The listing builds one solid part. Answer for the finished solid, in the listing's coordinates (mm). Coordinates: 2 decimals unless noted, no trailing zeros. Order: outer loops, then holes, each group sorted by start corner. A loop starts at its lowest first (then second) coordinate and runs counter-clockwise, first axis right, second up. Notation, with made-up numbers: (30.25, 54.5) - (81.25, 54.5) arc R17 cw to (81.25, 58.5) - close; hole circle Ø10 at (7.25, 23). An arc over 180 degrees is marked (long way). Use a Markdown table: item, result. Add a question column.
Item 1: The part is cut by section C-C, the plane x = 36. Give the vertices of the cut face in (y, z), then the cut area to 3 significant figures.
Item 2: The part is cut by section B-B, the plane x = 0. Give the vertices of the cut face in (y, z) (3 decimals).
Item 3: A flat-ended cylindrical pin translates along its axis: P1, Ø19, axis at x = 0, y = 0, coming from the -Z side. Find the tip coordinate at first contact, or state that the pin passes through.
Item 4: The part is cut by section A-A, the plane z = 0. Give the vertices of the cut face in (x, y), then the cut area to 3 significant figures.
Item 5: The part is cut by section D-D, the plane y = 20. Give the vertices of the cut face in (x, z), then the cut area to 3 significant figures.
Item 6: Find the intervals of material crossed by line 1 along X through (y, z) = (0, -55) (3 decimals); line 2 along Y through (x, z) = (36, 0); line 3 along Y through (x, z) = (0, 43) (3 decimals), in increasing order.
Item 7: The mould has two halves that part along Y. Classify faces 1 (the cylindrical face through (-2.07, 15.74, 48.41)), 2 (the flat face through (-50.8, -26, -1)), 3 (the flat face through (-1, 38.1, 18)): released by +Y, released by -Y, zero draft, split by the parting line, or undercut.
from build123d import *

# Parameters (mm, degrees)
F0_W     = 101.6
F0_H     = 152.4
F1_DEPTH = 38.1
F2_R     = 12.7
F3_DEPTH = 76.201
F4_R     = 25.4
F5_DEPTH = 101.601
F6_R     = 15.875
F7_DEPTH = 152.401


with BuildPart() as f1:
    # F0 (on Front) → F1 (new body, symmetric)
    with BuildSketch(Plane.XZ):
        Rectangle(F0_W, F0_H)
    extrude(amount=F1_DEPTH, both=True)

    # F2 (on face) → F3 (cut, through all)
    with BuildSketch(Plane.XZ.offset(38.1)):
        Circle(F2_R)
    extrude(amount=-F3_DEPTH, mode=Mode.SUBTRACT)

    # F4 (on face) → F5 (cut, through all)
    with BuildSketch(Plane.YZ.offset(50.8)):
        Circle(F4_R)
    extrude(amount=-F5_DEPTH, mode=Mode.SUBTRACT)

    # F6 (on face) → F7 (cut, through all)
    with BuildSketch(Plane.XY.offset(76.2)):
        Circle(F6_R)
    extrude(amount=-F7_DEPTH, mode=Mode.SUBTRACT)


solid = f1.part
Solution:
| question | item | result |
|---|---|---|
| 1 | outline | (-38.1, -76.2) - (38.1, -76.2) - (38.1, 76.2) - (-38.1, 76.2) - close; hole circle Ø50.8 at (0, 0) |
| 1 | area | 9,590 mm2 |
| 2 | outline | (-38.1, -76.2) - (-15.875, -76.2) - (-15.875, -19.828) arc R25.4 cw to (-21.997, -12.7) - (-38.1, -12.7) - close; (-38.1, 12.7) - (-21.997, 12.7) arc R25.4 cw to (-15.875, 19.828) - (-15.875, 76.2) - (-38.1, 76.2) - close; (15.875, -76.2) - (38.1, -76.2) - (38.1, -12.7) - (21.997, -12.7) arc R25.4 cw to (15.875, -19.828) - close; (15.875, 19.828) arc R25.4 cw to (21.997, 12.7) - (38.1, 12.7) - (38.1, 76.2) - (15.875, 76.2) - close |
| 3 | P1 | passes through |
| 4 | outline | (-50.8, -38.1) - (-12.7, -38.1) - (-12.7, -25.4) - (-50.8, -25.4) - close; (-50.8, 25.4) - (-12.7, 25.4) - (-12.7, 38.1) - (-50.8, 38.1) - close; (12.7, -38.1) - (50.8, -38.1) - (50.8, -25.4) - (12.7, -25.4) - close; (12.7, 25.4) - (50.8, 25.4) - (50.8, 38.1) - (12.7, 38.1) - close |
| 4 | area | 1,940 mm2 |
| 5 | outline | (-50.8, -76.2) - (50.8, -76.2) - (50.8, -15.66) - (-50.8, -15.66) - close; (-50.8, 15.66) - (50.8, 15.66) - (50.8, 76.2) - (-50.8, 76.2) - close |
| 5 | area | 12,300 mm2 |
| 6 | line 1 | x = -50.8 to -15.875, 15.875 to 50.8 |
| 6 | line 2 | y = -38.1 to -25.4, 25.4 to 38.1 |
| 6 | line 3 | y = -38.1 to -15.875, 15.875 to 38.1 |
| 7 | face 1 | undercut |
| 7 | face 2 | zero draft |
| 7 | face 3 | released by +Y |
